```python
from build123d import *

# Parameters (mm, degrees)
SKETCH1_R           = 50
SKETCH1_R_2         = 4
BOSS_EXTRUDE1_DEPTH = 5.63


with BuildPart() as part:
    # Sketch1 → Boss-Extrude1 (new body)
    with BuildSketch(Plane(origin=(0, 0, 0), x_dir=(1, 0, 0), z_dir=(0, 1, 0))):
        Polygon((0, 150), (200, 0), (0, -150), (-200, 0), align=None)
        with Locations(Location((0, 0, 0), (0, 0, 270))):
            Circle(SKETCH1_R, mode=Mode.SUBTRACT)
        with Locations(Location((170, 0, 0), (0, 0, 270))):
            Circle(SKETCH1_R_2, mode=Mode.SUBTRACT)
    extrude(amount=BOSS_EXTRUDE1_DEPTH)


solid = part.part
```
The listing builds one solid part. Answer for the finished solid, in the listing's coordinates (mm). Round coordinates to 2 decimals unless told otherwise and drop trailing zeros. Loops run counter-clockwise (first coordinate to the right, second up) from the corner with the lowest first, then second, coordinate; pieces in that order, holes last. Notation, with made-up numbers: (60.25, 34) - (107.25, 34) arc R5 cw to (107.25, 43) - close; hole circle Ø11 at (68, -27). An arc over 180 degrees is marked (long way). Return JSON: item names as keys, results as strings. Group by question number.
1. The part is cut by section C-C on x = 69. Determine the outline of the cut face in (y, z).
2. Consider probe 1 along X at (y, z) = (2.2, 0); probe 2 along Z at (x, y) = (-3, 5); probe 3 along X at (y, z) = (1.75, 1.5). Determine where each line is inside the solid, lowest interval first.
3. The part is cut by section D-D on z = -91.5. Determine the outline of the cut face in (x, y), then the cut area to 3 significant figures.
4. This flat-tipped pin is pushed along its axis until it touches: P1, Ø2, axis at x = 110.5, y = 2.5, coming from the -Z side (3 decimals). Where does it stop, or does it pass through?
5. The mould has two halves that part along X. Classify faces 1 (the flat face through (-101.4, 2.78, -73.95)), 2 (the cylindrical face through (173.966, 2.776, -0.521)), 3 (the flat face through (98.6, 2.78, -76.05)): pulls with the +X half, pulls with the -X half, needs draft (parallel to the pull), parting line crosses it, or undercut.
6. The part is cut by section A-A on y = 1.8. Determine the outline of the cut face in (x, z), then the cut area to 3 significant figures.
7. The part is cut by section B-B on x = -22. Determine the outline of the cut face in (y, z).
Resolved:
{
 "1": {"outline": "(0, -98.25) - (5.63, -98.25) - (5.63, 98.25) - (0, 98.25) - close"},
 "2": {"probe 1": "x = -200 to -50, 50 to 166, 174 to 200", "probe 2": "z = -147.75 to -49.91, 49.91 to 147.75", "probe 3": "x = -198 to -49.98, 49.98 to 166.29, 173.71 to 198"},
 "3": {"outline": "(-78, 0) - (78, 0) - (78, 5.63) - (-78, 5.63) - close", "area": "878 mm²"},
 "4": {"P1": "stops at z = -67.875"},
 "5": {"face 1": "pulls with the -X half", "face 2": "undercut", "face 3": "pulls with the +X half"},
 "6": {"outline": "(-200, 0) - (0, -150) - (200, 0) - (0, 150) - close; hole circle Ø100 at (0, 0); hole circle Ø8 at (170, 0)", "area": "52,100 mm²"},
 "7": {"outline": "(0, -133.5) - (5.63, -133.5) - (5.63, -44.9) - (0, -44.9) - close; (0, 44.9) - (5.63, 44.9) - (5.63, 133.5) - (0, 133.5) - close"}
}
